Autodesk Inventor part; units mm, degrees
ref_plane "Work Plane1" through (65, 0, 65) normal (1, 0, 0) x (0, 0, -1)
ref_plane "YZ Plane" through (0, 0, 0) normal (1, 0, 0) x (0, 1, 0)
ref_plane "XZ Plane" through (0, 0, 0) normal (0, 1, 0) x (-1, 0, 0)
sketch "Sketch1" plane through (0, 0, 0) normal (0, 1, 0) x (-1, 0, 0)
  line L0 (70, 0) -> (70, -70)
  line L1 (70, -70) -> (0, -70)
  line L2 (-70, 0) -> (-70, 70)
  line L3 (-70, 70) -> (0, 70)
  line L4 (0, 70) -> (70, 70)
  line L5 (70, 70) -> (70, 0)
  line L6 (0, -70) -> (-70, -70)
  line L7 (-70, -70) -> (-70, 0)
  point P0 (0, 0)
extrude "Extrusion1" add sketch "Sketch1" along normal blind 3
fillet "Fillet1" radius 5 3 edges at (70, 1.5, 70) (70, 1.5, -70) (-70, 1.5, 70)
fillet "Fillet2" radius 5 1 edges at (-70, 1.5, -70)
ref_plane "Work Plane1" through (65, 0, 65) normal (1, 0, 0) x (0, 0, -1)
sketch "Sketch6" plane through (70, 0, 65) normal (1, 0, 0) x (0, 0, -1)
  line L0 (65, 0) -> (57.2, 0)
  line L1 (130, 0) -> (0, 0)
  line L2 (65, 0) -> (72.8, 0)
  line L3 (57.2, 0) -> (57.2, -18)
  line L4 (72.8, 0) -> (72.8, -18)
  line L5 (65, 0) -> (65, -10)
  arc A0 (57.2, -18) -> (72.8, -18) centre (65, -10.2437) ccw
  line L6 (57.2, 0) -> (54.2, 0)
  line L7 (54.2, 0) -> (54.2, -18)
  line L8 (72.8, 0) -> (75.8, 0)
  line L9 (75.8, 0) -> (75.8, -18)
  arc A1 (54.2, -18) -> (75.8, -18) centre (65, -9.0916) ccw
  dimension "d17" = 18
  dimension "d21" = 3
  dimension "d22" = 3
extrude "Extrusion3" add sketch "Sketch6" against normal blind 18 contours L3 A0 L4 L1 L9 A1 L7
pattern_circular "Circular Pattern1" count 4 over 360 about axis through (0, -10, 0) along (0, 1, 0) of "Extrusion3"
sketch "Sketch8" plane through (0, 3, 0) normal (0, 1, 0) x (1, 0, 0)
  circle A0 centre (58.4636, -19.348) radius 2.5
  point P0 (0, 0)
  dimension "d35" = 5
extrude "Extrusion5" cut sketch "Sketch8" against normal blind 3
sketch "Sketch9" plane through (0, 3, 0) normal (0, 1, 0) x (1, 0, 0)
  circle A0 centre (-60.6489, 18.9578) radius 2.5
  point P0 (0, 0)
  dimension "d39" = 5
extrude "Extrusion6" cut sketch "Sketch9" against normal blind 3
sketch "Sketch10" plane through (0, 3, 0) normal (0, 1, 0) x (1, 0, 0)
  line L0 (70, -65) -> (70, 65)
  line L1 (70, 15.1257) -> (39.2687, 15.1257)
  line L2 (39.2687, 15.1257) -> (39.2687, -15.3197)
  line L3 (39.2687, -15.3197) -> (70, -15.3197)
  line L4 (70, -15.3197) -> (70, 15.1257)
  point P0 (0, 0)
extrude "Extrusion7" add sketch "Sketch10" along normal blind 10
sketch "Sketch11" plane through (0, 3, 0) normal (0, 1, 0) x (1, 0, 0)
  point P0 (0, 0)
sketch "Sketch12" plane through (0, 3, 0) normal (0, 1, 0) x (1, 0, 0)
  line L0 (39.2687, -15.3197) -> (39.2687, -70)
  line L1 (10.8, -70) -> (65, -70)
  line L2 (39.2687, -15.3197) -> (39.2687, 15.1257)
  line L3 (39.2687, -70) -> (-73.9803, -70)
  line L4 (-73.9803, -70) -> (-73.9803, 75.2408)
  line L5 (-73.9803, 75.2408) -> (39.2687, 75.2408)
  line L6 (39.2687, 75.2408) -> (39.2687, -70)
  point P0 (0, 0)
extrude "Extrusion8" cut sketch "Sketch12" against normal blind 100
sketch "Sketch13" plane through (0, 3, 0) normal (0, 1, 0) x (1, 0, 0)
  line L0 (39.2687, -15.3197) -> (74.5621, -15.3197)
  line L1 (74.5621, -15.3197) -> (74.5621, -76.2104)
  line L2 (74.5621, -76.2104) -> (39.2687, -76.2104)
  line L3 (39.2687, -76.2104) -> (39.2687, -15.3197)
  point P0 (0, 0)
extrude "Extrusion9" cut sketch "Sketch13" against normal blind 100
sketch "Sketch14" plane through (0, 3, 0) normal (0, 1, 0) x (1, 0, 0)
  line L0 (39.2687, 15.1257) -> (72.3919, 15.1257)
  line L1 (72.3919, 15.1257) -> (72.3919, 74.5163)
  line L2 (72.3919, 74.5163) -> (39.2687, 74.5163)
  line L3 (39.2687, 74.5163) -> (39.2687, 15.1257)
  point P0 (0, 0)
extrude "Extrusion10" cut sketch "Sketch14" against normal blind 100
sketch "Sketch17" plane through (70, -18, 10.8) normal (1, 0, 0) x (0, 0, -1)
  line L0 (-4.5197, 18) -> (-4.5197, 21)
  line L1 (-4.5197, 18) -> (-4.5197, 31)
  line L2 (-4.5197, 21) -> (25.9257, 21)
  line L3 (25.9257, 31) -> (25.9257, 18)
  line L4 (25.9257, 21) -> (-4.5197, 21)
  line L5 (-4.5197, 21) -> (-4.5197, 31)
  line L6 (-4.5197, 31) -> (25.9257, 31)
  line L7 (25.9257, 31) -> (25.9257, 21)
  point P0 (10.8, 18)
  dimension "d50" = 3
extrude "Extrusion11" cut sketch "Sketch17" against normal blind 100
sketch "Sketch18" plane through (39.2687, 0, -15.1257) normal (-1, 0, 0) x (0, 0, 1)
  line L0 (0, 3) -> (30.4454, 3)
  line L1 (30.4454, 3) -> (30.4454, 0)
  line L2 (30.4454, 0) -> (0, 0)
  line L3 (0, 0) -> (0, 3)
  point P0 (15.1257, 0)
extrude "Extrusion12" cut sketch "Sketch18" against normal blind 13
sketch "Sketch20" plane through (52, 0, 65) normal (-1, 0, 0) x (0, 0, 1)
  line L0 (-72.8, -18) -> (-72.8, 0)
  line L1 (-72.8, -9) -> (-57.2, -9)
  line L2 (-57.2, -18) -> (-57.2, 0)
  line L3 (-72.8, -18) -> (-72.8, -4)
  arc A0 (-72.8, -18) -> (-57.2, -18) centre (-65, -10.2437) ccw
  line L4 (-65, -21.2437) -> (-72.8, -21.2437)
  line L5 (-72.8, -4) -> (-72.8, -0.8)
  line L6 (-65, -21.2437) -> (-65, -3.2437)
  line L7 (-65, -21.2437) -> (-65, -11.2437)
  line L8 (-65, -11.2437) -> (-65, -1.2437)
  line L9 (-65, -1.2437) -> (-65, -0.8)
  arc A1 (-65, -0.8) -> (-72.6527, -4.1368) centre (-65, -11.2437) ccw
  arc A2 (-57.2, -4.2988) -> (-65, -0.8) centre (-65, -11.2437) ccw
  arc A3 (-72.6527, -4.1368) -> (-72.8, -4.2988) centre (-65, -11.2437) ccw
  arc A4 (-57.2, -4.2988) -> (-57.2, -4.2988) centre (-65, -11.2437) ccw
  line L10 (-72.8, -4.2988) -> (-72.8, 0)
  line L11 (-57.2, 0) -> (-57.2, -4.2988)
  line L12 (-57.2, 0) -> (-72.8, 0)
  line L13 (-57.2, -4.2988) -> (-57.2, 0)
  line L14 (-72.8, -4.2988) -> (-72.8, 0)
  line L15 (-72.8, 0) -> (-57.2, 0)
  point P0 (-65, 0)
  dimension "d55" = 14
  dimension "d56" = 3.2
  dimension "d57" = 18
  dimension "d58" = 10
  dimension "d59" = 10
extrude "Extrusion13" add sketch "Sketch20" against normal blind 18 contours L0 L12 L2 A2 A1 A3
sketch "Sketch22" plane through (52.2687, 0, 10.8) normal (0, 1, 0) x (1, 0, 0)
  line L0 (-0.2687, 21.6) -> (0, 21.6)
  line L1 (0, 21.6) -> (0, 0)
  line L2 (0, 0) -> (-0.2687, 0)
  line L3 (-0.2687, 0) -> (-0.2687, 21.6)
  point P0 (-52.2687, 10.8)
extrude "Extrusion14" add sketch "Sketch22" along normal blind 3
sketch "Sketch24" plane through (52.2687, 0, -15.1257) normal (-1, 0, 0) x (0, 0, 1)
  line L0 (30.4454, 3) -> (25.9257, 3)
  line L1 (25.9257, 3) -> (25.9257, 0)
  line L2 (25.9257, 0) -> (30.4454, 0)
  line L3 (30.4454, 0) -> (30.4454, 3)
  point P0 (15.1257, 0)
extrude "Extrusion16" add sketch "Sketch24" along normal blind 0.3
sketch "Sketch25" plane through (52.2687, 0, -15.1257) normal (-1, 0, 0) x (0, 0, 1)
  line L0 (0, 0) -> (4.3257, 0)
  line L1 (4.3257, 0) -> (4.3257, 3)
  line L2 (4.3257, 3) -> (0, 3)
  line L3 (0, 3) -> (0, 0)
  point P0 (15.1257, 0)
extrude "Extrusion17" add sketch "Sketch25" along normal blind 0.27
sketch "Sketch26" plane through (51.9687, 0, -15.1257) normal (-1, 0, 0) x (0, 0, 1)
  line L0 (30.4454, 3) -> (25.9257, 3)
  line L1 (25.9257, 3) -> (25.9257, 0)
  line L2 (25.9257, 0) -> (30.4454, 0)
  line L3 (30.4454, 0) -> (30.4454, 3)
  point P0 (15.1257, 0)
extrude "Extrusion18" cut sketch "Sketch26" against normal blind 0.03
sketch "Sketch27" plane through (70, 0, 15.3197) normal (0, 0, 1) x (1, 0, 0)
  line L0 (0, 3) -> (-18, 3)
  line L1 (-18, 3) -> (-18, 0)
  line L2 (-18, 0) -> (0, 0)
  line L3 (0, 0) -> (0, 3)
  point P0 (-70, 0)
extrude "Extrusion19" add sketch "Sketch27" along normal blind 3
sketch "Sketch32" plane through (51.9987, 0, -15.1257) normal (-1, 0, 0) x (0, 0, 1)
  line L0 (4.3257, 0) -> (-3, 0)
  line L1 (-3, 0) -> (-3, 3)
  line L2 (-3, 3) -> (4.3257, 3)
  line L3 (4.3257, 3) -> (4.3257, 0)
  point P0 (15.1257, 0)
extrude "Extrusion21" cut sketch "Sketch32" against normal blind 30
sketch "Sketch33" plane through (51.9987, 0, -15.1257) normal (-1, 0, 0) x (0, 0, 1)
  line L0 (33.4454, 0) -> (25.9257, 0)
  line L1 (25.9257, 3) -> (33.4257, 3)
  line L2 (33.4257, 3) -> (33.4257, 0)
  line L3 (33.4257, 0) -> (25.9257, 0)
  line L4 (25.9257, 0) -> (25.9257, 3)
  point P0 (15.1257, 0)
  dimension "d86" = 7.5
extrude "Extrusion22" add sketch "Sketch33" against normal blind 18
sketch "Sketch34" plane through (52, 3, -10.8) normal (0, 1, 0) x (1, 0, 0)
  line L0 (18, -29.1197) -> (18, -26.1197)
  line L1 (18, -29.1197) -> (18, -21.6)
  line L2 (18, -26.1197) -> (-0.0013, -26.1197)
  line L3 (-0.0013, -29.1) -> (-0.0013, -21.6)
  line L4 (-0.0013, -26.1197) -> (2.9987, -26.1197)
  line L5 (18, -26.1197) -> (15, -26.1197)
  circle A0 centre (15, -26.1197) radius 1.5
  circle A1 centre (2.9987, -26.1197) radius 1.5
  point P0 (-52, -10.8)
  dimension "d89" = 3
  dimension "d90" = 3
  dimension "d91" = 3
  dimension "d92" = 3
  dimension "d93" = 3
extrude "Extrusion23" cut sketch "Sketch34" against normal blind 18
sketch "Sketch35" plane through (70, -18, -10.8) normal (0, 0, -1) x (-1, 0, 0)
  line L0 (18, 21) -> (0, 21)
  line L1 (0, 21) -> (0, 18)
  line L2 (0, 18) -> (18, 18)
  line L3 (18, 18) -> (18, 21)
  point P0 (70, 18)
extrude "Extrusion24" add sketch "Sketch35" along normal blind 7.5
mirror "Mirror1" about plane through (0, 0, 0) normal (0, 0, 1) of "Extrusion23"
properties part number "smallpart"
Design review of the part built by this model. Coordinates are the model's own, in mm. A direction names the side the tool comes from. Round coordinates to 2 decimals unless told otherwise and drop trailing zeros. Order: outer loops, then holes, each group sorted by start corner. A loop starts at its lowest first (then second) coordinate and runs counter-clockwise, first axis right, second up. Notation, with made-up numbers: M 37.25,75 L 73.25,75 A8 cw 73.25,86 Z; hole C 66.25,84 d7. An arc over 180 degrees is marked long. Put each result on its own line as item: value.
Q1. Consider section D-D (x = 57.75). State the section outline as (y, z) points.
Reported:
outline: M -18,-10.8 L 0,-10.8 L 0,-18.3 L 3,-18.3 L 3,18.32 L 0,18.32 L 0,10.8 L -18,10.8 A14 ccw Z; hole M -18,-7.8 L -4.3,-7.8 A10.35 ccw -4.14,-7.65 A10.44 ccw -0.8,0 A10.44 ccw -4.3,7.8 L -18,7.8 A11 ccw Z
Q2. Machinability: for faces 5 (the face through (61.126, -21.243, 0.121)), 6 (the face through (68.386, 1.521, 15.894)), 7 (the face through (70, 0, -1)), 8 (the face through (61, 0, -14)), 9 (the face through (61, -9, 10.8)), which of the approach directions +Z, -Z, +X, -X, +Y, -Y give a long, thin tool a straight path to every point of the face, cutting with its end or side? Answer none if there is none.
Reported:
face 5: +X, -X
face 6: +Y, -Y
face 7: +Z, -Z, +X, +Y, -Y
face 8: -Z, +X, -X, -Y
face 9: +Z, +X, -X, -Y
Q3. Consider section C-C (z = -4.5). State the section outline as (x, y) points.
Reported:
outline: M 52,-22.35 L 70,-22.35 L 70,-20.28 L 52,-20.28 Z; M 52,-1.82 L 70,-1.82 L 70,3 L 52,3 Z
Q4. Insertion check: pin 1 Ø10 at (x, y) = (60.5, -16) entering from +Z; pin 2 Ø5.5 at (x, y) = (62, -8) entering from -Z; pin 3 Ø4 at (x, z) = (65, 16) entering from -Y. Each pin has a flat end and moves straight along its axis. Give the tip position at first contact, or say it passes through.
Reported:
pin 1: z = 10.8
pin 2: z = -10.8
pin 3: y = 0
Q5. Draft analysis for pull direction Z (two halves, no side actions). For faces 1 (the face through (61, 2, 18.32)), 2 (the face through (61, 3, 0)), 3 (the face through (61, -11, -7.8)), 4 (the face through (60.87, -1.74, 4.33)), state which applies: released by +Z, released by -Z, zero draft, split by the parting line, or undercut.
Reported:
face 1: released by +Z
face 2: zero draft
face 3: undercut
face 4: undercut
Q6. Consider section B-B (y = -20.75). State the section outline as (x, z) points, and give its area (3 significant figures).
Reported:
outline: M 52,-7.75 L 70,-7.75 L 70,-3.26 L 52,-3.26 Z; M 52,3.26 L 70,3.26 L 70,7.75 L 52,7.75 Z
area: 162 mm²
Q7. To check wall thickness, follow line 1 (Z direction, x = 67, y = 1); line 2 (Z direction, x = 59.5, y = -13.25); line 3 (Y direction, x = 59.75, z = 0). State the ranges of each line that lie inside material, in increasing order.
Reported:
line 1: -18.3 to -16.82, -13.82 to 13.82, 16.82 to 18.32
line 2: -10.8 to -7.8, 7.8 to 10.8
line 3: -23.09 to -21.24, -0.8 to 3
Q8. Consider section A-A (x = 67). State the section outline as (y, z) points, and give its area (3 significant figures).
Reported:
outline: M -18,-10.8 L 0,-10.8 L 0,-13.82 L 3,-13.82 L 3,13.82 L 0,13.82 L 0,10.8 L -18,10.8 A14 ccw Z; M 0,-18.3 L 3,-18.3 L 3,-16.82 L 0,-16.82 Z; M 0,16.82 L 3,16.82 L 3,18.32 L 0,18.32 Z; hole M -18,-7.8 L -4.3,-7.8 A10.35 ccw -4.14,-7.65 A10.44 ccw -0.8,0 A10.44 ccw -4.3,7.8 L -18,7.8 A11 ccw Z
area: 271 mm²
